Geometry: final body of the model. Coordinates: model frame, mm. A direction names the side the tool comes from. Give positions to 0.01 mm unless a question says otherwise; leave off trailing zeros. Write each loop counter-clockwise with the first axis right and the second up, starting at its lowest first coordinate (ties: lowest second). Pieces come first, ordered by that corner, then holes.
Autodesk Inventor part; units mm, degrees
ref_plane "YZ Plane" through (0, 0, 0) normal (1, 0, 0) x (0, 1, 0)
ref_plane "XZ Plane" through (0, 0, 0) normal (0, 1, 0) x (-1, 0, 0)
ref_plane "XY Plane" through (0, 0, 0) normal (0, 0, 1) x (1, 0, 0)
sketch "Skizze1" plane through (0, 0, 0) normal (0, 1, 0) x (-1, 0, 0)
  line L0 (17, 1) -> (22, 1)
  line L1 (22, 1) -> (22, 0)
  line L2 (22, 0) -> (0, 0)
  line L3 (0, 12.5) -> (0, 0)
  line L4 (99.15, 0) -> (-16.525, 0)
  line L5 (0, -2.5) -> (0, 15)
  line L6 (16, 12.5) -> (0, 12.5)
  arc A0 (16, 12.5) -> (17, 1) centre (82.625, 12.5) ccw
  line L7 (16, 12.5) -> (16, 0) construction
  dimension "d5" = 44
  dimension "d6" = 12.5
  dimension "d7" = 1
  dimension "d15" = 16
  dimension "d16" = 17
revolve "Umdrehung1" add sketch "Skizze1" angle 360 about axis through (0, 0, 12.5) along (0, 0, -1)
sketch "Skizze3" plane through (0, 0, 12.5) normal (0, 0, 1) x (1, 0, 0)
  circle A0 centre (0, 0) radius 22
  circle A1 centre (0, 0) radius 5.075
  dimension "d8" = 10.15
extrude "Extrusion2" cut sketch "Skizze3" against normal through all contours A1
sketch "Skizze4" plane through (0, 0, 12.5) normal (0, 0, 1) x (1, 0, 0)
  circle A0 centre (0, 0) radius 5.075
  circle A1 centre (0, 0) radius 16
  line L0 (-7.5, -7.5) -> (7.5, -7.5)
  line L1 (7.5, -7.5) -> (7.5, 7.5)
  line L2 (7.5, 7.5) -> (-7.5, 7.5)
  line L3 (-7.5, 7.5) -> (-7.5, -7.5)
  line L4 (-7.5, -7.5) -> (7.5, 7.5) construction
  line L5 (7.5, -7.5) -> (-7.5, 7.5) construction
  dimension "d11" = 15
  dimension "d12" = 15
extrude "Extrusion3" add sketch "Skizze4" along normal blind 14.7 contours L3 L2 L1 L0
properties part number "Seil_Rolle_Antrieb_Links" material "PC/ABS-Kunststoff"
Item 1: Section A-A, the plane x = 0. Return the cut outline in (y, z) (3 decimals).
Found:
outline: (-22, 0) - (-5.075, 0) - (-5.075, 27.2) - (-7.5, 27.2) - (-7.5, 12.5) - (-16, 12.5) arc R66.625 cw to (-17, 1) - (-22, 1) - close; (5.075, 0) - (22, 0) - (22, 1) - (17, 1) arc R66.625 cw to (16, 12.5) - (7.5, 12.5) - (7.5, 27.2) - (5.075, 27.2) - close
Item 2: Section C-C, the plane z = 21.25. Return the cut outline in (x, y) (3 decimals), plus the area to 3 significant figures.
Found:
outline: (-7.5, -7.5) - (7.5, -7.5) - (7.5, 7.5) - (-7.5, 7.5) - close; hole circle Ø10.15 at (0, 0)
area: 144 mm2
Item 3: Pull-direction query (Y, two-part tool) for faces 4 (the face through (-4.027, -3.088, 13.79)), 5 (the face through (-10, 0, 12.5)), 6 (the face through (0, -7.5, 20)); classes: +Y half, -Y half, draft (parallel to the pull), parting line (faces both ways), or undercut.
Found:
face 4: undercut
face 5: draft
face 6: -Y half
Item 4: Line query: L1, parallel to Y at x = 0, z = 14.25 (3 decimals); L2, parallel to Y at x = 0, z = 9.75 (3 decimals); L3, parallel to Z at x = -16.5, y = 9. Output: solid intervals per line, ascending.
Found:
L1: y = -7.5 to -5.075, 5.075 to 7.5
L2: y = -16.057 to -5.075, 5.075 to 16.057
L3: z = 0 to 1
Item 5: Pin query (flat end, axial travel): pin 1 Ø7.5 at (y, z) = (3.5, 20.5) entering from +X; pin 2 Ø2 at (y, z) = (7.5, 16) entering from -X; pin 3 Ø12 at (x, z) = (6.5, 15) entering from -Y; pin 4 Ø2 at (x, y) = (-1, -12) entering from -Z. Return the tip coordinate at first contact, or that it passes through.
Found:
pin 1: stops at x = 7.5
pin 2: stops at x = -7.5
pin 3: stops at y = -15.97
pin 4: stops at z = 0
Item 6: Section D-D, the plane z = 8.75. Return the cut outline in (x, y) (3 decimals).
Found:
outline: circle Ø32.211 at (0, 0); hole circle Ø10.15 at (0, 0)
Item 7: Reachability of faces 1 (the face through (-7.5, 0, 20)), 2 (the face through (-11.3, -12.93, 1)), 3 (the face through (0, 7.5, 20)) from +Z, -Z, +X, -X, +Y, -Y: full face, straight path, thin tool, end or side. Return the list, or none.
Found:
face 1: +Z, -X, +Y, -Y
face 2: +Z
face 3: +Z, +X, -X, +Y
